```python
from build123d import *

# Parameters (mm, degrees)
SKETCH1_R           = 22.5
BOSS_EXTRUDE1_DEPTH = 3.5
SKETCH2_R           = 9
SKETCH2_R_2         = 9.000000000000007
CUT_EXTRUDE1_DEPTH  = 33.58066911528982
SKETCH7_R           = 5
CUT_EXTRUDE2_DEPTH  = 33.58066911528982
SKETCH8_R           = 5
BOSS_EXTRUDE2_DEPTH = 5
BOSS_EXTRUDE4_START = -5
BOSS_EXTRUDE4_DEPTH = 5
CUT_EXTRUDE3_DEPTH  = 7
BOSS_EXTRUDE8_START = 5
SKETCH15_R          = 22.5
SKETCH15_R_2        = 4.5
SKETCH15_R_3        = 5
BOSS_EXTRUDE8_DEPTH = 5


with BuildPart() as part:
    # Sketch1 → Boss-Extrude1 (new, symmetric)
    with BuildSketch(Plane(origin=(0, 0, 0), x_dir=(1, 0, 0), z_dir=(0, 1, 0))):
        with Locations(Location((0, 0, 0), (0, 0, 270))):
            Circle(SKETCH1_R)
    extrude(amount=BOSS_EXTRUDE1_DEPTH, both=True)

    # Sketch2 → Cut-Extrude1 (cut, through all)
    with BuildSketch(Plane(origin=(0, 3.5, 0), x_dir=(1, 0, 0), z_dir=(0, 1, 0))):
        with Locations((4.245e-14, 15.5)):
            Circle(SKETCH2_R)
        with Locations((13.42339375865983, -7.749999999999429)):
            Circle(SKETCH2_R_2)
        with Locations((-13.423393758657767, -7.7500000000005755)):
            Circle(SKETCH2_R)
    extrude(amount=-CUT_EXTRUDE1_DEPTH, mode=Mode.SUBTRACT)

    # Sketch7 → Cut-Extrude2 (cut, through all)
    with BuildSketch(Plane(origin=(0, 3.5, 0), x_dir=(1, 0, 0), z_dir=(0, 1, 0))):
        with Locations(Location((0, 0, 0), (0, 0, 270))):
            Circle(SKETCH7_R)
    extrude(amount=-CUT_EXTRUDE2_DEPTH, mode=Mode.SUBTRACT)

    # Sketch8 → Boss-Extrude2 (add)
    with BuildSketch(Plane.XZ.offset(3.5)):
        with BuildLine():
            ThreePointArc((8.634046628681784, -18.040322580645523), (16.921597628085173, -10.661122535323484), (20, -4.9e-15))
            ThreePointArc((20, 0), (19.985094686202057, 0.7720041344048885), (19.940400961646176, 1.5428575724221159))
            ThreePointArc((19.94040096164584, 1.542857572422255), (5.629165124599421, 3.250000000000214), (11.30635433296457, 16.497465008220495))
            ThreePointArc((11.306354332964553, 16.497465008220313), (1.07592e-12, 20), (-11.306354332962771, 16.497465008221535))
            ThreePointArc((-11.30635433296279, 16.497465008221706), (-5.629165124598033, 3.250000000000197), (-19.940400961645828, 1.5428575724255662))
            ThreePointArc((-19.940400961645913, 1.542857572425538), (-17.320508075688895, -9.999999999999787), (-8.634046628681693, -18.040322580645565))
            ThreePointArc((-8.634046628682263, -18.04032258064596), (1.954e-14, -6.5000000000000036), (8.634046628682352, -18.04032258064592))
        make_face()
        with Locations(Location((0, 0, 0), (0, 0, 90))):
            Circle(SKETCH8_R, mode=Mode.SUBTRACT)
    extrude(amount=BOSS_EXTRUDE2_DEPTH)

    # Sketch9 → Boss-Extrude4 (add)
    with BuildSketch(Plane.XZ.offset(8.5).offset(BOSS_EXTRUDE4_START)):
        with BuildLine():
            Line((-16.681897360151837, 4.646428786213113), (-19.940400961645906, 1.5428575724256501))
            ThreePointArc((-19.940400961645906, 1.5428575724256497), (-5.6291651245981145, 3.250000000000062), (-11.306354332962595, 16.497465008221653))
            Line((-11.306354332962595, 16.497465008221656), (-12.364874045810183, 12.123732504111118))
            ThreePointArc((-12.364874045810181, 12.123732504111118), (-9.52627944162794, 5.50000000000032), (-16.681897360151837, 4.646428786213113))
        make_face()
        with BuildLine():
            Line((12.3648740458121, 12.123732504109935), (11.306354332964363, 16.49746500822045))
            ThreePointArc((11.306354332964363, 16.49746500822045), (5.629165124599578, 3.249999999999936), (19.940400961646137, 1.5428575724225722))
            Line((19.94040096164614, 1.5428575724225757), (16.681897360152977, 4.646428786211002))
            ThreePointArc((16.681897360152977, 4.6464287862110005), (9.526279441629708, 5.499999999999686), (12.3648740458121, 12.123732504109935))
        make_face()
    extrude(amount=BOSS_EXTRUDE4_DEPTH)

    # Sketch10 → Cut-Extrude3 (cut)
    with BuildSketch(Plane(origin=(0, 3.5, 0), x_dir=(1, 0, 0), z_dir=(0, 1, 0))):
        with BuildLine():
            ThreePointArc((-6.73691741017109, 21.467741935483897), (2.481e-14, 6.5), (6.736917410171204, 21.46774193548386))
            ThreePointArc((6.736917410171204, 21.46774193548386), (19.485571585149323, 11.250000000000961), (21.96006858310362, -4.899529347333845))
            ThreePointArc((21.96006858310362, -4.899529347333845), (5.629165124599583, -3.24999999999993), (15.223151172932472, -16.56821258814737))
            ThreePointArc((15.223151172932472, -16.56821258814737), (6.8083e-13, -22.500000000000007), (-15.223151172931468, -16.568212588148292))
            ThreePointArc((-15.223151172931468, -16.568212588148292), (-5.629165124598114, -3.2500000000000657), (-21.960068583102636, -4.899529347338252))
            ThreePointArc((-21.960068583102636, -4.899529347338252), (-19.485571585150417, 11.249999999999057), (-6.73691741017109, 21.467741935483897))
        make_face()
    extrude(amount=-CUT_EXTRUDE3_DEPTH, mode=Mode.SUBTRACT)

    # Sketch15 → Boss-Extrude8 (add)
    # profile 1 of 2: a face of its own
    with BuildSketch(Plane(origin=(0, -3.5000000000000004, 0), x_dir=(1, 0, 0), z_dir=(0, 1, 0)).offset(BOSS_EXTRUDE8_START)):
        with Locations(Location((0, 0, 0), (0, 0, 270))):
            Circle(SKETCH15_R)
        with BuildLine():
            Line((-11.306354332962597, -16.49746500822166), (-12.364874045810184, -12.12373250411112))
            ThreePointArc((-12.364874045810184, -12.123732504111118), (-17.32050807568759, -10.000000000000831), (-16.681897360151837, -4.646428786213116))
            Line((-16.681897360151837, -4.646428786213116), (-19.9404009616459, -1.5428575724256433))
            ThreePointArc((-19.940400961645906, -1.5428575724256435), (-17.320508075689144, 9.99999999999936), (-8.63404662868249, 18.04032258064519))
            ThreePointArc((-8.634046628682489, 18.040322580645185), (1.865e-14, 6.499999999999998), (8.634046628682592, 18.040322580645135))
            ThreePointArc((8.634046628682588, 18.04032258064514), (17.320508075688394, 10.000000000000643), (19.94040096164614, -1.5428575724225746))
            Line((19.94040096164614, -1.5428575724225748), (16.681897360152977, -4.646428786211005))
            ThreePointArc((16.68189736015298, -4.646428786211002), (17.601507340572077, -6.078663140883227), (17.923393758659827, -7.749999999999429))
            ThreePointArc((17.923393758659827, -7.74999999999943), (16.206077830934763, -11.286476969231293), (12.3648740458121, -12.123732504109933))
            Line((12.3648740458121, -12.123732504109936), (11.306354332964357, -16.49746500822045))
            ThreePointArc((11.30635433296436, -16.49746500822045), (1.06937e-12, -20), (-11.306354332962597, -16.49746500822166))
        make_face(mode=Mode.SUBTRACT)
        with Locations(Location((4.245e-14, 15.5, 0), (0, 0, 270))):
            Circle(SKETCH15_R_2, mode=Mode.SUBTRACT)
    # profile 2 of 2: a face of its own
    with BuildSketch(Plane(origin=(0, -3.5000000000000004, 0), x_dir=(1, 0, 0), z_dir=(0, 1, 0)).offset(BOSS_EXTRUDE8_START)):
        with BuildLine():
            Line((-19.9404009616459, -1.5428575724256433), (-16.681897360151837, -4.646428786213116))
            ThreePointArc((-16.681897360151837, -4.646428786213116), (-9.526279441627942, -5.5000000000003215), (-12.364874045810184, -12.12373250411112))
            Line((-12.364874045810184, -12.12373250411112), (-11.306354332962597, -16.49746500822166))
            ThreePointArc((-11.306354332962597, -16.49746500822166), (1.06704e-12, -20.000000000000004), (11.306354332964357, -16.49746500822045))
            Line((11.306354332964357, -16.49746500822045), (12.3648740458121, -12.123732504109936))
            ThreePointArc((12.3648740458121, -12.123732504109936), (9.526279441629708, -5.499999999999686), (16.681897360152977, -4.646428786211005))
            Line((16.681897360152977, -4.646428786211005), (19.94040096164614, -1.5428575724225746))
            ThreePointArc((19.94040096164614, -1.5428575724225746), (17.3205080756884, 10.000000000000643), (8.634046628682588, 18.04032258064514))
            ThreePointArc((8.634046628682588, 18.04032258064514), (1.902e-14, 6.5), (-8.63404662868249, 18.040322580645185))
            ThreePointArc((-8.63404662868249, 18.040322580645185), (-17.320508075689144, 9.99999999999936), (-19.9404009616459, -1.5428575724256433))
        make_face()
        with Locations(Location((0, 0, 0), (0, 0, 270))):
            Circle(SKETCH15_R_3, mode=Mode.SUBTRACT)
    extrude(amount=-BOSS_EXTRUDE8_DEPTH)


solid = part.part
```
Verification items for the finished model (mm, model axes). A direction names the side the tool comes from. Coordinates: 2 decimals unless noted, no trailing zeros. Write each loop counter-clockwise with the first axis right and the second up, starting at its lowest first coordinate (ties: lowest second). Pieces come first, ordered by that corner, then holes. Notation, with made-up numbers: (72, 35) - (99, 35) arc R17 ccw to (99, 40) - close; hole circle Ø4 at (61.5, 2). An arc over 180 degrees is marked (long way). Write item = value, one per line.
Q1. Cross-section at B-B (y = -4.75). Enter the section's corners in (x, z), plus the area to 3 significant figures.
Answer:
outline = (-19.94, 1.54) arc R20 ccw to (-8.63, -18.04) arc R9 cw (long way) to (8.63, -18.04) arc R20 ccw to (19.94, 1.54) - (16.68, 4.65) arc R4.5 cw (long way) to (12.36, 12.12) - (11.31, 16.5) arc R20 ccw to (-11.31, 16.5) - (-12.36, 12.12) arc R4.5 cw (long way) to (-16.68, 4.65) - close; hole circle Ø10 at (0, 0)
area = 818 mm²
Q2. Material ranges on L1, parallel to X at y = -0.95, z = 0; L2, parallel to X at y = -2, z = 7.75; L3, parallel to Z at x = 3.5, y = -5.75, recorded low to high. Write a range as from..to.
Answer:
L1 = -22.5..-5, 5..22.5
L2 = -21.12..-17.92, -8.92..8.92, 17.92..21.12
L3 = -7.21..-3.57, 3.57..19.69
Q3. Cross-section at D-D (z = 7.75). Enter the section's corners in (x, y).
Answer:
outline = (-21.12, -3.5) - (-17.92, -3.5) - (-17.92, 1.5) - (-21.12, 1.5) - close; (-8.92, -8.5) - (8.92, -8.5) - (8.92, 1.5) - (-8.92, 1.5) - close; (17.92, -3.5) - (21.12, -3.5) - (21.12, 1.5) - (17.92, 1.5) - close
Q4. Cross-section at A-A (z = 0). Enter the section's corners in (x, y).
Answer:
outline = (-22.5, -3.5) - (-20, -3.5) - (-20, -8.5) - (-5, -8.5) - (-5, 1.5) - (-22.5, 1.5) - close; (5, -8.5) - (20, -8.5) - (20, -3.5) - (22.5, -3.5) - (22.5, 1.5) - (5, 1.5) - close
Q5. Access from +Z, -Z, +X, -X, +Y, -Y to the whole of each face (thin tool, end or side, straight path). Record for faces 1 (the face through (0, -6, 20)), 2 (the face through (11.843, -5.965, 14.28)), 3 (the face through (-0.234, -5.965, -6.503)).
Answer:
face_1 = +Z, -Y
face_2 = +Z, +X, -Y
face_3 = -Y
Q6. Cross-section at C-C (x = 0). Enter the section's corners in (y, z), plus the area to 4 significant figures.
Answer:
outline = (-8.5, -6.5) - (-3.5, -6.5) - (-3.5, -11) - (1.5, -11) - (1.5, -5) - (-8.5, -5) - close; (-8.5, 5) - (1.5, 5) - (1.5, 22.5) - (-3.5, 22.5) - (-3.5, 20) - (-8.5, 20) - close; (-3.5, -22.5) - (1.5, -22.5) - (1.5, -20) - (-3.5, -20) - close
area = 212.5 mm²
Q7. Go/stop test with flat-tipped pins: pin 1 Ø1 at (x, y) = (-12.5, -4.5) entering from -Z; pin 2 Ø5 at (x, z) = (-4.5, -13.5) entering from -Y; pin 3 Ø1 at (y, z) = (-1, 0) entering from +X. Record where each tip stops, or that it passes through.
Answer:
pin_1 = -16
pin_2 = -3.5
pin_3 = 22.5
Q8. Mould release check, pull along X, two halves, no side actions. Record for faces 4 (the face through (9.69, -2.32, 5.24)), 5 (the face through (18.334, -5.965, 3.073)), 6 (the face through (-11.83, -5.96, 14.34)): released by +X, released by -X, zero draft, split by the parting line, or undercut.
Answer:
face_4 = undercut
face_5 = released by +X
face_6 = released by -X
